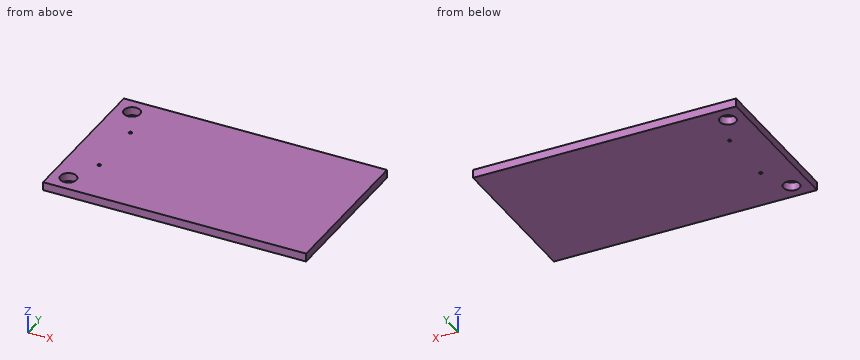
from build123d import *

# Parameters (mm, degrees)
SKETCH1_W           = 50
SKETCH1_H           = 30
SKETCH1_R           = 1.524
SKETCH1_R_2         = 0.3
BOSS_EXTRUDE1_DEPTH = 1.58


with BuildPart() as part:
    # Sketch1 → Boss-Extrude1 (new body)
    with BuildSketch(Plane.XY):
        Rectangle(SKETCH1_W, SKETCH1_H)
        with Locations(Location((-21.8, 11.8, 0), (0, 0, 180))):
            Circle(SKETCH1_R, mode=Mode.SUBTRACT)
        with Locations(Location((-21.8, -11.8, 0), (0, 0, 180))):
            Circle(SKETCH1_R, mode=Mode.SUBTRACT)
        with Locations((-19.032, 5.8)):
            Circle(SKETCH1_R_2, mode=Mode.SUBTRACT)
        with Locations((-19.032, -5.8)):
            Circle(SKETCH1_R_2, mode=Mode.SUBTRACT)
    extrude(amount=BOSS_EXTRUDE1_DEPTH)


solid = part.part
The listing builds one solid part. Answer for the finished solid, in the listing's coordinates (mm). Coordinates: 2 decimals unless noted, no trailing zeros. Write each loop counter-clockwise with the first axis right and the second up, starting at its lowest first coordinate (ties: lowest second). Pieces come first, ordered by that corner, then holes. Notation, with made-up numbers: (-18.75, 87) - (16.25, 87) arc R7 cw to (16.25, 97) - close; hole circle Ø11 at (30.5, 49). An arc over 180 degrees is marked (long way). Put each result on its own line as item: value.
1. Find the intervals of material crossed by line 1 along Y through (x, z) = (-21.8, 0.6); line 2 along X through (y, z) = (11.8, 0.8), in increasing order. Write a range as from..to.
Answer sheet:
line 1: y = -15..-13.32, -10.28..10.28, 13.32..15
line 2: x = -25..-23.32, -20.28..25
2. The part is cut by section B-B on x = -21.8. Give the vertices of the cut face in (y, z).
Answer sheet:
outline: (-15, 0) - (-13.32, 0) - (-13.32, 1.58) - (-15, 1.58) - close; (-10.28, 0) - (10.28, 0) - (10.28, 1.58) - (-10.28, 1.58) - close; (13.32, 0) - (15, 0) - (15, 1.58) - (13.32, 1.58) - close
3. The part is cut by section A-A on y = 11.8. Give the vertices of the cut face in (x, z), plus the area to 3 significant figures.
Answer sheet:
outline: (-25, 0) - (-23.32, 0) - (-23.32, 1.58) - (-25, 1.58) - close; (-20.28, 0) - (25, 0) - (25, 1.58) - (-20.28, 1.58) - close
area: 74.2 mm^2
4. The part is cut by section C-C on y = -10.75. Give the vertices of the cut face in (x, z).
Answer sheet:
outline: (-25, 0) - (-22.9, 0) - (-22.9, 1.58) - (-25, 1.58) - close; (-20.7, 0) - (25, 0) - (25, 1.58) - (-20.7, 1.58) - close
